Print and shaded views of the part. All mm, measured from the part's lowest x, y and z. A direction names the side the tool comes from. Give positions to 0.01 mm unless a question says otherwise; leave off trailing zeros. Write each loop counter-clockwise with the first axis right and the second up, starting at its lowest first coordinate (ties: lowest second). Pieces come first, ordered by that corner, then holes. Notation, with made-up numbers: M 1,4 L 19,4 A22 cw 19,10 Z; hole C 32,-14.5 d10. An arc over 180 degrees is marked long. One line per question, with ' | ' between items. Start each with the question number.
1. Flat gauge pins, fed straight in: pin 1 (8 mm diameter, centred on y = 32.5, z = 9.5, fed in from -X); pin 2 (1 mm diameter, centred on y = 90, z = 27.5, fed in from -X); pin 3 (4 mm diameter, centred on x = 114.3, y = 68.326, fed in from +Z). Where does each tip first touch, or does it go through?
2. Cut at A-A, the plane y = 88.9. Write the cut outline in (x, z).
3. Wall check: L1, parallel to Y at x = 114.3, z = 24.75; L2, parallel to X at y = 68, z = 32; L3, parallel to X at y = 11.5, z = 6. Give the ranges that are in metal, low to high.
4. Cut at D-D, the plane y = 39.5. Write the cut outline in (x, z).
5. Which spindle directions (+Z, -Z, +X, -X, +Y, -Y) get a long thin tool onto all of the face, cutting with end or side? Do the marked faces 1, 2 and 3. Say none if no direction does.
6. Cut at B-B, the plane z = 9. Write the cut outline in (x, y).
7. Cut at C-C, the plane x = 142. Write the cut outline in (y, z), then the cut area to 3 significant figures.
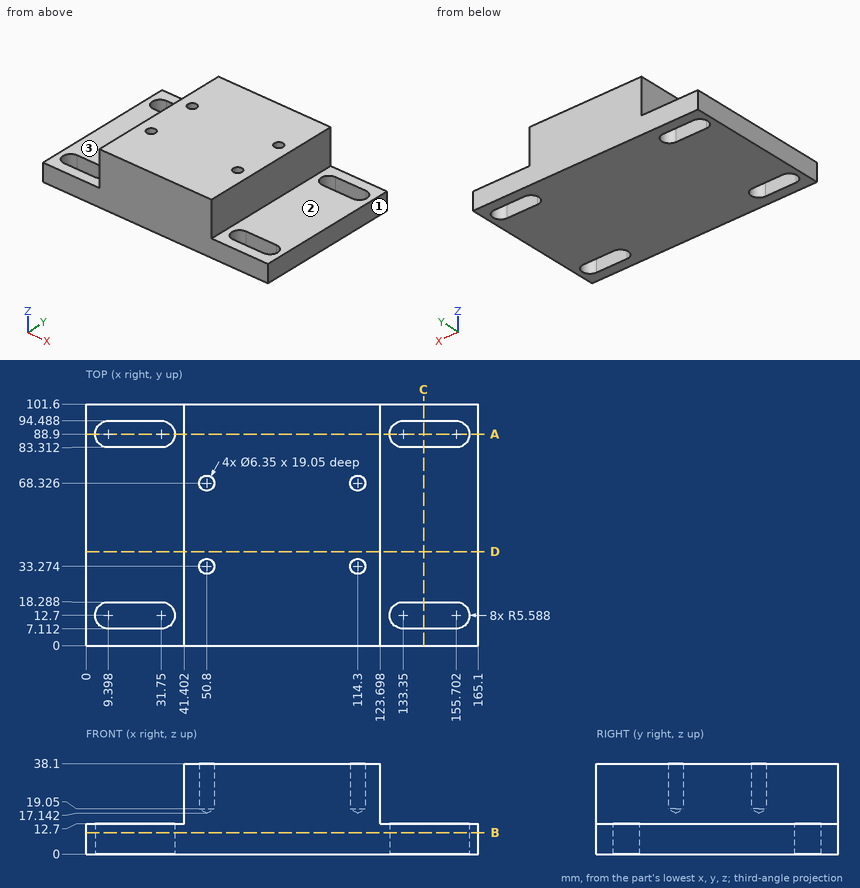
Here are the results:
1) pin 1: x = 0 | pin 2: x = 41.4 | pin 3: z = 18.34
2) outline: M 0,0 L 3.81,0 L 3.81,12.7 L 0,12.7 Z; M 37.34,0 L 127.76,0 L 127.76,12.7 L 123.7,12.7 L 123.7,38.1 L 41.4,38.1 L 41.4,12.7 L 37.34,12.7 Z; M 161.29,0 L 165.1,0 L 165.1,12.7 L 161.29,12.7 Z
3) L1: 0 to 30.1, 36.45 to 65.15, 71.5 to 101.6 | L2: 41.4 to 47.64, 53.96 to 111.14, 117.46 to 123.7 | L3: 0 to 3.94, 37.21 to 127.89, 161.16 to 165.1
4) outline: M 0,0 L 165.1,0 L 165.1,12.7 L 123.7,12.7 L 123.7,38.1 L 41.4,38.1 L 41.4,12.7 L 0,12.7 Z
5) face 1: +Z, -Z, +X, +Y, -Y | face 2: +Z, +X, +Y, -Y | face 3: +Z, -X, +Y, -Y
6) outline: M 0,0 L 165.1,0 L 165.1,101.6 L 0,101.6 Z; hole M 9.4,7.11 L 31.75,7.11 A5.59 ccw 31.75,18.29 L 9.4,18.29 A5.59 ccw Z; hole M 9.4,83.31 L 31.75,83.31 A5.59 ccw 31.75,94.49 L 9.4,94.49 A5.59 ccw Z; hole M 133.35,7.11 L 155.7,7.11 A5.59 ccw 155.7,18.29 L 133.35,18.29 A5.59 ccw Z; hole M 133.35,83.31 L 155.7,83.31 A5.59 ccw 155.7,94.49 L 133.35,94.49 A5.59 ccw Z
7) outline: M 0,0 L 7.11,0 L 7.11,12.7 L 0,12.7 Z; M 18.29,0 L 83.31,0 L 83.31,12.7 L 18.29,12.7 Z; M 94.49,0 L 101.6,0 L 101.6,12.7 L 94.49,12.7 Z | area: 1,010 mm^2
